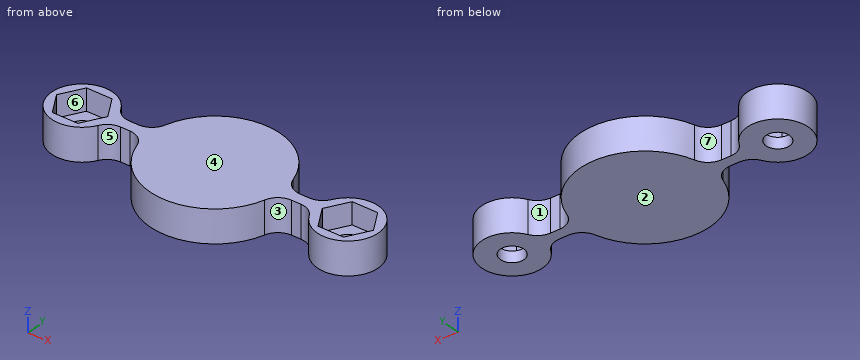
```python
from build123d import *

# Parameters (mm, degrees)
F1_DEPTH = 4.7625
F2_R     = 5.08
F4_DEPTH = 6.35
F5_R     = 3.429
F6_DEPTH = 9.526


with BuildPart() as f1:
    # F0 (on Top) → F1 (new body, symmetric)
    with BuildSketch(Plane.XY):
        with BuildLine():
            Line((-29.352889, -1.5875), (-18.983739, -1.5875))
            ThreePointArc((-18.983739, -1.5875), (0, -19.05), (18.983739, -1.5875))
            Line((18.983739, -1.5875), (29.352889, -1.5875))
            ThreePointArc((29.352889, -1.5875), (46.99, 0), (29.352889, 1.5875))
            Line((29.352889, 1.5875), (18.983739, 1.5875))
            ThreePointArc((18.983739, 1.5875), (0, 19.05), (-18.983739, 1.5875))
            Line((-18.983739, 1.5875), (-29.352889, 1.5875))
            ThreePointArc((-29.352889, 1.5875), (-46.99, 0), (-29.352889, -1.5875))
        make_face()
    extrude(amount=F1_DEPTH, both=True)

    # F2
    f2_edges = [f1.edges().sort_by_distance(p)[0] for p in [
        (-29.352889, 1.5875, 0),
        (18.983739, 1.5875, 0),
        (-18.983739, 1.5875, 0),
        (29.352889, 1.5875, 0),
        (29.352889, -1.5875, 0),
        (-18.983739, -1.5875, 0),
        (-29.352889, -1.5875, 0),
        (18.983739, -1.5875, 0),
    ]]
    fillet(f2_edges, radius=F2_R)

    # F3 (on face) → F4 (cut)
    with BuildSketch(Plane.XY.offset(4.7625)):
        Polygon((-30.767652, 0), (-34.433826, 6.35), (-41.766174, 6.35), (-45.432348, 0), (-41.766174, -6.35), (-34.433826, -6.35), align=None)
        Polygon((41.766174, -6.35), (45.432348, 0), (41.766174, 6.35), (34.433826, 6.35), (30.767652, 0), (34.433826, -6.35), align=None)
    extrude(amount=-F4_DEPTH, mode=Mode.SUBTRACT)

    # F5 (on face) → F6 (cut, through all)
    with BuildSketch(Plane(origin=(0, 0, -4.7625), x_dir=(1, 0, 0), z_dir=(0, 0, -1))):
        with Locations((-38.1, 0)):
            Circle(F5_R)
        with Locations((38.1, 0)):
            Circle(F5_R)
    extrude(amount=-F6_DEPTH, mode=Mode.SUBTRACT)


solid = f1.part
```
The listing builds one solid part. Answer for the finished solid, in the listing's coordinates (mm). Face numbers are marked on the shaded views. A direction names the side the tool comes from. Coordinates: 2 decimals unless noted, no trailing zeros. Write each loop counter-clockwise with the first axis right and the second up, starting at its lowest first coordinate (ties: lowest second). Pieces come first, ordered by that corner, then holes. Notation, with made-up numbers: (20, -34.5) -> (34, -34.5) arc R19 ccw to (34, -3.5) -> close; hole circle Ø8 at (52, 12.25). An arc over 180 degrees is marked (long way). Write each question's results on one line, items separated by ' | '. Start each with the question number.
1) A cutting plane is placed at B-B (x = -38.5). Determine the outline of the cut face in (y, z).
2) A cutting plane is placed at C-C (x = 38.1). Determine the outline of the cut face in (y, z).
3) Flat-ended cylindrical pins translate along their axes: pin 1 Ø2 at (x, z) = (24, -0.5) entering from -Y; pin 2 Ø1.3 at (x, z) = (24.5, 0) entering from +Y; pin 3 Ø2 at (y, z) = (8, 2.5) entering from -X. Find the tip coordinate at first contact, or state that the pin passes through.
4) A cutting plane is placed at D-D (y = 16.5). Determine the outline of the cut face in (x, z).
5) For a pull along X with two mould halves and no side action, classify the marked faces 1, 2 and 3 as +X half, -X half, draft (parallel to the pull), parting line (faces both ways), or undercut.
6) A tool of negligible diameter and unlimited length cuts with its end or side. For the marked faces 4, 5, 6 and 7, from which of +Z, -Z, +X, -X, +Y, -Y can it reach the whole face along a straight path? Write none if from no direction.
7) Straight lines are drawn through the part: probe 1 along X at (y, z) = (0, -2.2); probe 2 along Y at (x, z) = (-38.1, -3.5); probe 3 along X at (y, z) = (6.5, -2.5). For each, find the intervals that lie inside material, in ascending order.
8) A cutting plane is placed at A-A (z = 0.75). Determine the outline of the cut face in (x, y), then the cut area to 3 significant figures.
Values follow:
1) outline: (-8.88, -4.76) -> (-3.41, -4.76) -> (-3.41, -1.59) -> (-6.35, -1.59) -> (-6.35, 4.76) -> (-8.88, 4.76) -> close; (3.41, -4.76) -> (8.88, -4.76) -> (8.88, 4.76) -> (6.35, 4.76) -> (6.35, -1.59) -> (3.41, -1.59) -> close
2) outline: (-8.89, -4.76) -> (-3.43, -4.76) -> (-3.43, -1.59) -> (-6.35, -1.59) -> (-6.35, 4.76) -> (-8.89, 4.76) -> close; (3.43, -4.76) -> (8.89, -4.76) -> (8.89, 4.76) -> (6.35, 4.76) -> (6.35, -1.59) -> (3.43, -1.59) -> close
3) pin 1: y = -1.59 | pin 2: y = 1.59 | pin 3: x = -43.58
4) outline: (-9.52, -4.76) -> (9.52, -4.76) -> (9.52, 4.76) -> (-9.52, 4.76) -> close
5) face 1: undercut | face 2: draft | face 3: undercut
6) face 4: +Z, +X, -X, +Y, -Y | face 5: +Z, -Z, -Y | face 6: +Z | face 7: +Z, -Z, +Y
7) probe 1: -46.99 to -41.53, -34.67 to 34.67, 41.53 to 46.99 | probe 2: -8.89 to -3.43, 3.43 to 8.89 | probe 3: -44.16 to -32.04, -17.91 to 17.91, 32.04 to 44.16
8) outline: (-30.29, -4.24) arc R5.08 cw to (-25.82, -1.59) -> (-23.19, -1.59) arc R5.08 cw to (-18.31, -5.26) arc R19.05 ccw to (18.31, -5.26) arc R5.08 cw to (23.19, -1.59) -> (25.82, -1.59) arc R5.08 cw to (30.29, -4.24) arc R8.89 ccw (long way) to (30.29, 4.24) arc R5.08 cw to (25.82, 1.59) -> (23.19, 1.59) arc R5.08 cw to (18.31, 5.26) arc R19.05 ccw to (-18.31, 5.26) arc R5.08 cw to (-23.19, 1.59) -> (-25.82, 1.59) arc R5.08 cw to (-30.29, 4.24) arc R8.89 ccw (long way) to start; hole (-45.43, 0) -> (-41.77, -6.35) -> (-34.43, -6.35) -> (-30.77, 0) -> (-34.43, 6.35) -> (-41.77, 6.35) -> close; hole (30.77, 0) -> (34.43, -6.35) -> (41.77, -6.35) -> (45.43, 0) -> (41.77, 6.35) -> (34.43, 6.35) -> close | area: 1,440 mm²
